from build123d import *

# Parameters (mm, degrees)
F2_W     = 20
F2_H     = 12
F3_DEPTH = 8


with BuildPart() as f1:
    # F0 (on Front) → F1 (revolve)
    with BuildSketch(Plane.XZ):
        Polygon((-3.375, 0), (0, 0), (0, 78.4805588418), (-2, 78.4805588418), (-2, 56.99), (-6, 56.99), (-6, 44.99), (-8, 44.99), (-8, 41.29), (-6, 41.29), (-6, 35.29), (-8, 35.29), (-8, 28.29), (-11.15, 28.29), (-11.15, 2.29), (-3.375, 2.29), align=None)
    revolve(axis=Axis((0, 0, 37.5557746226), (0, 0, 1)))

    # F2 (on Front) → F3 (join, symmetric)
    with BuildSketch(Plane.XZ):
        with Locations((1.5, -6)):
            Rectangle(F2_W, F2_H)
    extrude(amount=F3_DEPTH, both=True)


solid = f1.part
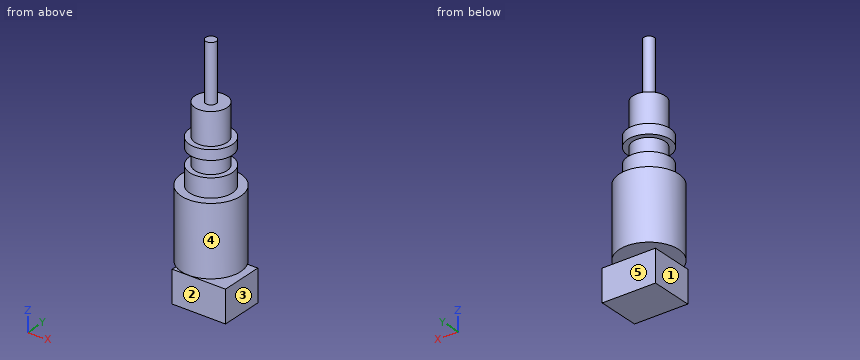
Verification items for the finished model (mm, model axes). Face numbers are marked on the shaded views. A direction names the side the tool comes from. Coordinates: 2 decimals unless noted, no trailing zeros. Order: outer loops, then holes, each group sorted by start corner. A loop starts at its lowest first (then second) coordinate and runs counter-clockwise, first axis right, second up. Notation, with made-up numbers: M 28,-37.5 L 47,-37.5 A36 ccw 47,0.5 Z; hole C -15.5,44.25 d8. An arc over 180 degrees is marked long. One line per item, written item: value. Start each with the question number.
Item 1: Depth check by flat-ended pin: P1, Ø5, axis at x = -2.5, y = -0.5, coming from the +Z side; P2, Ø8, axis at y = -0.5, z = 33.5, coming from the +X side; P3, Ø3.5, axis at y = -2, z = -5, coming from the -X side; P4, Ø6, axis at x = -3, z = -6.5, coming from the +Y side. Enter the tip coordinate at first touch or a pass-through.
Item 2: Access from +Z, -Z, +X, -X, +Y, -Y to the whole of each face (thin tool, end or side, straight path). Record for the marked faces 1, 2, 3, 4 and 5.
Item 3: Sectioned sample at C-C on z = 15. Record the cut outline in (x, y), then the cut area to 3 significant figures.
Item 4: Sectioned sample at B-B on y = 5. Record the cut outline in (x, z) (3 decimals).
Item 5: Thickness scan on probe 1 along Z at (x, y) = (-7.5, -1); probe 2 along Z at (x, y) = (-8.25, -1.5); probe 3 along Z at (x, y) = (0.75, -4.75). Record the ranges inside material, lowest first.
Calculated:
1. P1: z = 78.48
1. P2: x = 8
1. P3: x = -8.5
1. P4: y = 8
2. face 1: -Z, -X, +Y, -Y
2. face 2: -Z, +X, -X, -Y
2. face 3: +Z, -Z, +X, +Y, -Y
2. face 4: +Z
2. face 5: -Z, +X, -X, +Y
3. outline: C 0,0 d22.3
3. area: 391 mm^2
4. outline: M -9.966,2.29 L 9.966,2.29 L 9.966,28.29 L 6.245,28.29 L 6.245,35.29 L 3.317,35.29 L 3.317,41.29 L 6.245,41.29 L 6.245,44.99 L 3.317,44.99 L 3.317,56.99 L -3.317,56.99 L -3.317,44.99 L -6.245,44.99 L -6.245,41.29 L -3.317,41.29 L -3.317,35.29 L -6.245,35.29 L -6.245,28.29 L -9.966,28.29 Z; M -8.5,-12 L 11.5,-12 L 11.5,0 L -8.5,0 Z
5. probe 1: -12 to 0, 2.29 to 35.29, 41.29 to 44.99
5. probe 2: -12 to 0, 2.29 to 28.29
5. probe 3: -12 to 0, 2.29 to 56.99
